Design review of the part built by this model. Coordinates are the model's own, in mm. A direction names the side the tool comes from. Coordinates: 2 decimals unless noted, no trailing zeros. Write each loop counter-clockwise with the first axis right and the second up, starting at its lowest first coordinate (ties: lowest second). Pieces come first, ordered by that corner, then holes. Notation, with made-up numbers: (-13, 78) - (15, 78) arc R28 ccw to (15, 114) - close; hole circle Ø4 at (59.25, 39). An arc over 180 degrees is marked (long way). Use a Markdown table: item, result.
Autodesk Inventor part; units mm, degrees
ref_plane "YZ Plane" through (0, 0, 0) normal (1, 0, 0) x (0, 1, 0)
ref_plane "XZ Plane" through (0, 0, 0) normal (0, 1, 0) x (-1, 0, 0)
ref_plane "XY Plane" through (0, 0, 0) normal (0, 0, 1) x (1, 0, 0)
sketch "Sketch1" plane through (0, 0, 0) normal (0, 0, 1) x (1, 0, 0)
  line L0 (0, 0) -> (15, 0)
  line L1 (15, 0) -> (15, 3)
  line L2 (15, 3) -> (0, 3)
  line L3 (0, 3) -> (0, 0)
  circle A0 centre (0, 2.5) radius 2.5
  point P0 (0, 1.5)
  point P1 (2.4495, 3)
  point P2 (2.4495, 3)
  dimension "d0" = 15
  dimension "d1" = 3
  dimension "d2" = 5
extrude "Extrusion1" add sketch "Sketch1" against normal blind 30
ref_plane "Work Plane1" through (0, 0, -20) normal (0, 0, 1) x (1, 0, 0)
sketch "Sketch2" plane through (0, 0, -20) normal (0, 0, 1) x (1, 0, 0)
  arc A0 (2.4495, 3) -> (0, 0) centre (0, 2.5) ccw
  circle A1 centre (0, 2.5) radius 2.51
  dimension "d6" = 5.02
extrude "Extrusion2" cut sketch "Sketch2" along normal blind 10
properties part number "Clip2" material "Stainless Steel"
(1) Take a section at C-C on x = 12. Write out the cut boundary in (y, z), and give its area (3 significant figures).
Determined:
| item | result |
|---|---|
| outline | (0, -30) - (3, -30) - (3, 0) - (0, 0) - close |
| area | 90.0 mm2 |
(2) Take a section at A-A on y = 2.5. Write out the cut boundary in (x, z), and give its area (3 significant figures).
Determined:
| item | result |
|---|---|
| outline | (-2.5, -30) - (15, -30) - (15, 0) - (-2.5, 0) - (-2.5, -10) - (2.51, -10) - (2.51, -20) - (-2.5, -20) - close |
| area | 475 mm2 |
(3) Take a section at B-B on y = 4.55. Write out the cut boundary in (x, z), and give its area (3 significant figures).
Determined:
| item | result |
|---|---|
| outline | (-1.43, -30) - (1.43, -30) - (1.43, -20) - (-1.43, -20) - close; (-1.43, -10) - (1.43, -10) - (1.43, 0) - (-1.43, 0) - close |
| area | 57.2 mm2 |
(4) Draft analysis for pull direction Z (two halves, no side actions). For faces 4 (the cylindrical face through (-2, 4, -25)), 5 (the flat face through (6, 2, 0)), 6 (the flat face through (0, 3, -20)), state which applies: +Z half, -Z half, draft (parallel to the pull), parting line (faces both ways), or undercut.
Determined:
| item | result |
|---|---|
| face 4 | draft |
| face 5 | +Z half |
| face 6 | undercut |
(5) For L1, parallel to Z at x = -1, y = 2.05; L2, parallel to Y at x = 4.75, z = -24.25; L3, parallel to X at y = 2.35, z = -5.5, list the stretches that pass through material, from the lowest coordinate up. Write a range as from..to.
Determined:
| item | result |
|---|---|
| L1 | -30..-20, -10..0 |
| L2 | 0..3 |
| L3 | -2.5..15 |
(6) Machinability: for faces 1 (the flat face through (9, 3, -15)), 2 (the flat face through (6, 2, -30)), 3 (the cylindrical face through (2.03, 1.024, -15.07)), which of the approach directions +Z, -Z, +X, -X, +Y, -Y give a long, thin tool a straight path to every point of the face, cutting with its end or side? Answer none if there is none.
Determined:
| item | result |
|---|---|
| face 1 | +Z, -Z, +X, +Y |
| face 2 | -Z, +X, -X, +Y, -Y |
| face 3 | -X |
(7) Take a section at D-D on z = -7.5. Write out the cut boundary in (x, y), and give its area (3 significant figures).
Determined:
| item | result |
|---|---|
| outline | (0, 0) - (15, 0) - (15, 3) - (2.45, 3) arc R2.5 ccw (long way) to start |
| area | 58.5 mm2 |
(8) For pin 1 (4 mm diameter, centred on x = 9.5, z = -8.5, fed in from +Y), flat-tipped, find the tip position at first contact; note if it passes through.
Determined:
| item | result |
|---|---|
| pin 1 | y = 3 |
